Could you check a few things on this model? Use its own coordinates, in mm. A direction names the side the tool comes from. Give positions to 0.01 mm unless a question says otherwise; leave off trailing zeros. Loops run counter-clockwise (first coordinate to the right, second up) from the corner with the lowest first, then second, coordinate; pieces in that order, holes last. Notation, with made-up numbers: M -21,79.25 L -11,79.25 A9 cw -11,90.25 Z; hole C 31.5,77.25 d10. An arc over 180 degrees is marked long. Answer in a Markdown table with one row per item. Add a question column.
1. Thinking about a two-plate mould opening in Y: for faces 4 (the flat face through (10, -25, 25)), 5 (the flat face through (20, -5, 0)), 6 (the cylindrical face through (9.86, -53.173, 0.705)), which applies, released by +Y, released by -Y, zero draft, split by the parting line, or undercut?
2. I'm going to push flat-ended pins straight in: pin 1 Ø6 at (x, z) = (9, 47) entering from -Y; pin 2 Ø3 at (x, z) = (13.5, 22.5) entering from -Y; pin 3 Ø6 at (x, z) = (7, 37.5) entering from -Y. Where does each tip first touch, or does it pass through?
3. If we section it at A-A on z = 0: List the corners of the cut face in (x, y) for me (3 decimals).
4. If we section it at B-B on y = -64: List the corners of the cut face in (x, z) for me.
5. I need wall thicknesses on line 1 along Z through (x, y) = (19.25, -17); line 2 along X through (y, z) = (64, 2.75); line 3 along Y through (x, z) = (4.5, -50). Which ranges of each line are inside material? Lowest first, please. Write a range as from..to.
6. If we section it at D-D on y = 38: List the corners of the cut face in (x, z) for me.
7. Which directions (+Z, -Z, +X, -X, +Y, -Y) give clear straight access to the entire face, cutting with the end or side of a thin tool? Please do faces 1 (the flat face through (12, 0, -15)), 2 (the flat face through (10, -7.5, 59)), 3 (the flat face through (10, 75, 0)).
```python
from build123d import *

# Parameters (mm, degrees)
SKETCH1_W               = 50
SKETCH1_H               = 50
SKETCH1_R               = 1.7
BOSS_EXTRUDE1_DEPTH     = 20
CUT_EXTRUDE1_START      = -12.5
SKETCH2_R               = 2.65
SKETCH2_R_2             = 1.7
CUT_EXTRUDE1_DEPTH      = 12.5
BOSS_EXTRUDE3_DEPTH     = 20
SKETCH5_W               = 4
SKETCH5_H               = 10
SKETCH5_W_2             = 10
SKETCH5_H_2             = 4
CUT_EXTRUDE2_DEPTH      = 8
CHAMFER1_START          = -5
CHAMFER1_DEPTH          = 10
CHAMFER1_START_2        = -17.720633844
CHAMFER1_2_OUTLINE_W    = 8
CHAMFER1_2_OUTLINE_H    = 10
CHAMFER1_2_DEPTH        = 5.441267688
CHAMFER1_START_3        = 12.279366156
CHAMFER1_3_OUTLINE_W    = 8
CHAMFER1_3_OUTLINE_H    = 10
CHAMFER1_3_DEPTH        = 5.441267688
CHAMFER1_4_DEPTH        = 10
CUT_EXTRUDE4_DEPTH      = 108.935165725
CUT_EXTRUDE4_DEPTH_BACK = 108.935165725
SKETCH7_R               = 3.25
SKETCH8_R               = 3.2
CUT_EXTRUDE5_DEPTH      = 114.275107592
CIRPATTERN1_COUNT       = 4
SKETCH9_R               = 1.35
CUT_EXTRUDE6_DEPTH      = 15
CIRPATTERN2_COUNT       = 4


with BuildPart() as part:
    # Sketch1 → Boss-Extrude1 (new body)
    with BuildSketch(Plane(origin=(0, 0, 0), x_dir=(0, 0, -1), z_dir=(1, 0, 0))):
        Rectangle(SKETCH1_W, SKETCH1_H)
        with Locations((-19, 19)):
            Circle(SKETCH1_R, mode=Mode.SUBTRACT)
        with Locations((19, 19)):
            Circle(SKETCH1_R, mode=Mode.SUBTRACT)
        with Locations((19, -19)):
            Circle(SKETCH1_R, mode=Mode.SUBTRACT)
        with Locations((-19, -19)):
            Circle(SKETCH1_R, mode=Mode.SUBTRACT)
    extrude(amount=BOSS_EXTRUDE1_DEPTH)

    # Sketch2 → Cut-Extrude1 (cut)
    # profile 1 of 4: a face of its own
    with BuildSketch(Plane(origin=(20, 0, 0), x_dir=(0, 0, -1), z_dir=(1, 0, 0)).offset(CUT_EXTRUDE1_START)):
        with Locations((-19, 19)):
            Circle(SKETCH2_R)
        with Locations((-19, 19)):
            Circle(SKETCH2_R_2, mode=Mode.SUBTRACT)
    # profile 2 of 4: a face of its own
    with BuildSketch(Plane(origin=(20, 0, 0), x_dir=(0, 0, -1), z_dir=(1, 0, 0)).offset(CUT_EXTRUDE1_START)):
        with Locations((19, 19)):
            Circle(SKETCH2_R)
        with Locations((19, 19)):
            Circle(SKETCH2_R_2, mode=Mode.SUBTRACT)
    # profile 3 of 4: a face of its own
    with BuildSketch(Plane(origin=(20, 0, 0), x_dir=(0, 0, -1), z_dir=(1, 0, 0)).offset(CUT_EXTRUDE1_START)):
        with Locations((19, -19)):
            Circle(SKETCH2_R)
        with Locations((19, -19)):
            Circle(SKETCH2_R_2, mode=Mode.SUBTRACT)
    # profile 4 of 4: a face of its own
    with BuildSketch(Plane(origin=(20, 0, 0), x_dir=(0, 0, -1), z_dir=(1, 0, 0)).offset(CUT_EXTRUDE1_START)):
        with Locations((-19, -19)):
            Circle(SKETCH2_R)
        with Locations((-19, -19)):
            Circle(SKETCH2_R_2, mode=Mode.SUBTRACT)
    extrude(amount=CUT_EXTRUDE1_DEPTH, mode=Mode.SUBTRACT)

    # Sketch3 → Cut-Revolve1 (revolve, cut)
    with BuildSketch(Plane(origin=(0, 0, 0), x_dir=(1, 0, 0), z_dir=(0, 1, 0))):
        with BuildLine():
            Line((0, 0), (0, 15.125))
            ThreePointArc((0, 15.125), (10.694990065, 10.694990065), (15.125, 0))
            Line((15.125, 0), (0, 0))
        make_face()
    revolve(axis=Axis((-993.762626263, 0, 0), (1, 0, 0)), mode=Mode.SUBTRACT)

    # Sketch4 → Boss-Extrude3 (add)
    with BuildSketch(Plane(origin=(20, 0, 0), x_dir=(0, 0, -1), z_dir=(1, 0, 0))):
        Polygon((42.5, 7.5), (25, 25), (25, -25), (42.5, -7.5), (75, -7.5), (75, 7.5), align=None)
        Polygon((-25, 25), (25, 25), (7.5, 42.5), (7.5, 75), (-7.5, 75), (-7.5, 42.5), align=None)
        Polygon((7.5, -42.5), (25, -25), (-25, -25), (-7.5, -42.5), (-7.5, -75), (7.5, -75), align=None)
        Polygon((-25, -25), (-25, 25), (-42.5, 7.5), (-75, 7.5), (-75, -7.5), (-42.5, -7.5), align=None)
    extrude(amount=-BOSS_EXTRUDE3_DEPTH)

    # Sketch5 → Cut-Extrude2 (cut)
    with BuildSketch(Plane(origin=(20, 0, 0), x_dir=(0, 0, -1), z_dir=(1, 0, 0))):
        with Locations((15, 0)):
            Rectangle(SKETCH5_W, SKETCH5_H)
        with Locations((0, 15)):
            Rectangle(SKETCH5_W_2, SKETCH5_H_2)
        with Locations((0, -15)):
            Rectangle(SKETCH5_W_2, SKETCH5_H_2)
        with Locations((-15, 0)):
            Rectangle(SKETCH5_W, SKETCH5_H)
    extrude(amount=-CUT_EXTRUDE2_DEPTH, mode=Mode.SUBTRACT)

    # Chamfer1: read off the stored shape, not the designer's step
    # Chamfer1 outline → Chamfer1 (cut)
    with BuildSketch(Plane(origin=(0, 0, 0), x_dir=(1, 0, 0), z_dir=(0, 1, 0)).offset(CHAMFER1_START)):
        Polygon((12, 12.279366156), (20, 12), (20, 13), (12, 13), align=None)
        Polygon((12, -17), (12, -17.720633844), (20, -18), (20, -17), align=None)
        Polygon((12, -12.279366156), (12, -13), (20, -13), (20, -12), align=None)
        Polygon((12, 17), (20, 17), (20, 18), (12, 17.720633844), align=None)
    extrude(amount=CHAMFER1_DEPTH, mode=Mode.SUBTRACT)

    # Chamfer1 2 outline → Chamfer1 2 (cut)
    with BuildSketch(Plane(origin=(0, 0, 0), x_dir=(1, 0, 0), z_dir=(0, 1, 0)).offset(CHAMFER1_START_2)):
        with Locations((16, 0)):
            Rectangle(CHAMFER1_2_OUTLINE_W, CHAMFER1_2_OUTLINE_H)
    extrude(amount=CHAMFER1_2_DEPTH, mode=Mode.SUBTRACT)

    # Chamfer1 3 outline → Chamfer1 3 (cut)
    with BuildSketch(Plane(origin=(0, 0, 0), x_dir=(1, 0, 0), z_dir=(0, 1, 0)).offset(CHAMFER1_START_3)):
        with Locations((16, 0)):
            Rectangle(CHAMFER1_3_OUTLINE_W, CHAMFER1_3_OUTLINE_H)
    extrude(amount=CHAMFER1_3_DEPTH, mode=Mode.SUBTRACT)

    # Chamfer1 4 outline → Chamfer1 4 (cut)
    with BuildSketch(Plane.XY.offset(CHAMFER1_START)):
        Polygon((12, 17.720633844), (20, 17.720633844), (20, 18), align=None)
        Polygon((12, 12.279366156), (20, 12), (20, 12.279366156), align=None)
        Polygon((20, -18), (20, -17.720633844), (12, -17.720633844), align=None)
        Polygon((20, -12), (12, -12.279366156), (20, -12.279366156), align=None)
    extrude(amount=CHAMFER1_4_DEPTH, mode=Mode.SUBTRACT)

    # Sketch7 → Cut-Extrude4 (cut, two sides: drawn at the far end of the back side and taken through both)
    with BuildSketch(Plane(origin=(20, 0, 0), x_dir=(0, 0, -1), z_dir=(1, 0, 0)).offset(-CUT_EXTRUDE4_DEPTH_BACK)):
        with Locations((50, 0)):
            Circle(SKETCH7_R)
        with Locations((0, -50)):
            Circle(SKETCH7_R)
        with Locations((-50, 0)):
            Circle(SKETCH7_R)
        with Locations((0, 50)):
            Circle(SKETCH7_R)
    extrude(amount=CUT_EXTRUDE4_DEPTH + CUT_EXTRUDE4_DEPTH_BACK, mode=Mode.SUBTRACT)

    # Sketch8 → Cut-Extrude5 (cut, symmetric)
    with BuildSketch(Plane.XZ.offset(7.5)):
        with Locations(Location((10, -64, 0), (0, 0, 270))):
            Circle(SKETCH8_R)
    cut_extrude5 = extrude(amount=CUT_EXTRUDE5_DEPTH, both=True, mode=Mode.SUBTRACT)

    # CirPattern1: Cut-Extrude5 ×4 about axis
    cirpattern1_axis = Axis((20, 0, 0), (1, 0, 0))
    for i in range(1, CIRPATTERN1_COUNT):
        add(cut_extrude5.rotate(cirpattern1_axis, i * 360 / CIRPATTERN1_COUNT), mode=Mode.SUBTRACT)

    # Sketch9 → Cut-Extrude6 (cut)
    with BuildSketch(Plane(origin=(0, -25, -25), x_dir=(1, 0, 0), z_dir=(0, -0.7071067811865438, -0.7071067811865513))):
        with Locations(Location((15, 10, 0), (0, 0, 270))):
            Circle(SKETCH9_R)
        with Locations(Location((15, -10, 0), (0, 0, 270))):
            Circle(SKETCH9_R)
    cut_extrude6 = extrude(amount=-CUT_EXTRUDE6_DEPTH, mode=Mode.SUBTRACT)

    # CirPattern2: Cut-Extrude6 ×4 about axis
    cirpattern2_axis = Axis((0, 0, 0), (1, 0, 0))
    for i in range(1, CIRPATTERN2_COUNT):
        add(cut_extrude6.rotate(cirpattern2_axis, i * 360 / CIRPATTERN2_COUNT), mode=Mode.SUBTRACT)


solid = part.part
```
Results:
| question | item | result |
|---|---|---|
| 1 | face 4 | released by -Y |
| 1 | face 5 | zero draft |
| 1 | face 6 | undercut |
| 2 | pin 1 | y = -7.5 |
| 2 | pin 2 | y = -29 |
| 2 | pin 3 | y = -15.5 |
| 3 | outline | M 0,-75 L 20,-75 L 20,-53.25 L 0,-53.25 Z; M 0,-46.75 L 20,-46.75 L 20,-18 L 12,-17.721 L 12,-12.279 L 20,-12 L 20,12 L 12,12.279 L 12,17.721 L 20,18 L 20,46.75 L 0,46.75 L 0,15.125 A15.125 cw 0,-15.125 Z; M 0,53.25 L 20,53.25 L 20,75 L 0,75 Z; hole C 10,-64 d6.4; hole C 10,64 d6.4 |
| 4 | outline | M 0,-7.5 L 6.8,-7.5 L 6.8,7.5 L 0,7.5 Z; M 13.2,-7.5 L 20,-7.5 L 20,7.5 L 13.2,7.5 Z |
| 5 | line 1 | -33..-20.74, -17.26..-5, 5..17.26, 20.74..33 |
| 5 | line 2 | 0..6.8, 13.2..20 |
| 5 | line 3 | -7.5..-3.25, 3.25..7.5 |
| 6 | outline | M 0,-12 L 20,-12 L 20,12 L 0,12 Z |
| 7 | face 1 | +X |
| 7 | face 2 | +Z, +X, -X, -Y |
| 7 | face 3 | +Z, -Z, +X, -X, +Y |
